Part model, mm, in its own coordinate system. Round coordinates to 2 decimals unless told otherwise and drop trailing zeros. Loops run counter-clockwise (first coordinate to the right, second up) from the corner with the lowest first, then second, coordinate; pieces in that order, holes last.
(1) Flat gauge pin, fed straight in: pin 1 (2.5 mm diameter, centred on x = 17.14, z = 43.28, fed in from +Y). Where does the tip first touch, or does it go through?
(2) Cut at C-C on y = 2.75. List the corners of the cut face in (x, z).
(3) Cut at B-B on x = 20. List the corners of the cut face in (y, z).
(4) Cut at A-A on z = 25. List the corners of the cut face in (x, y), then the cut area to 3 significant figures.
(5) Mould opens along X. For faces 1 (the face through (33, 2, 0)), 2 (the face through (0, 2, 25)), 3 (the face through (18.73, 2.03, 42.06)) say: +X half, -X half, draft (parallel to the pull), parting line (faces both ways), or undercut.
(6) Probe probe 1 along X at (y, z) = (2.9, 25); probe 2 along Z at (x, y) = (21.5, 0.7); probe 3 along X at (y, z) = (3.4, 26). List the from-to ranges inside material, lowest first.
from build123d import *

# Parameters (mm, degrees)
BOSS_EXTRUDE1_DEPTH = 50
SKETCH3_R           = 4
CUT_EXTRUDE1_DEPTH  = 10
SKETCH4_W           = 25
SKETCH4_H           = 50
CUT_EXTRUDE2_DEPTH  = 10
SKETCH6_R           = 2
CUT_EXTRUDE4_DEPTH  = 83.1035931


with BuildPart() as part:
    # Sketch2 → Boss-Extrude1 (new body)
    with BuildSketch(Plane.XY):
        Polygon((4, 4), (90, 4), (90, 0), (0, 0), (0, 4), align=None)
    extrude(amount=BOSS_EXTRUDE1_DEPTH)

    # Sketch3 → Cut-Extrude1 (cut)
    with BuildSketch(Plane(origin=(0, 4, 0), x_dir=(1, 0, 0), z_dir=(0, 1, 0))):
        with Locations(Location((20, -25, 0), (0, 0, 270))):
            Circle(SKETCH3_R)
    extrude(amount=-CUT_EXTRUDE1_DEPTH, mode=Mode.SUBTRACT)

    # Sketch4 → Cut-Extrude2 (cut)
    with BuildSketch(Plane(origin=(0, 4, 0), x_dir=(1, 0, 0), z_dir=(0, 1, 0))):
        with Locations((77.5, -25)):
            Rectangle(SKETCH4_W, SKETCH4_H)
    extrude(amount=-CUT_EXTRUDE2_DEPTH, mode=Mode.SUBTRACT)

    # Sketch6 → Cut-Extrude4 (cut, through all)
    with BuildSketch(Plane(origin=(0, 4, 0), x_dir=(1, 0, 0), z_dir=(0, 1, 0))):
        with Locations(Location((17.143662574, -43.278165567, 0), (0, 0, 180))):
            Circle(SKETCH6_R)
        with Locations(Location((22.856337427, -6.721834433, 0), (0, 0, 180))):
            Circle(SKETCH6_R)
    extrude(amount=-CUT_EXTRUDE4_DEPTH, mode=Mode.SUBTRACT)


solid = part.part
Final values:
1. pin 1: passes through
2. outline: (0, 0) - (65, 0) - (65, 50) - (0, 50) - close; hole circle Ø4 at (17.14, 43.28); hole circle Ø8 at (20, 25); hole circle Ø4 at (22.86, 6.72)
3. outline: (0, 0) - (4, 0) - (4, 21) - (0, 21) - close; (0, 29) - (4, 29) - (4, 50) - (0, 50) - close
4. outline: (0, 0) - (16, 0) - (16, 4) - (0, 4) - close; (24, 0) - (65, 0) - (65, 4) - (24, 4) - close
4. area: 228 mm2
5. face 1: draft
5. face 2: -X half
5. face 3: undercut
6. probe 1: x = 0 to 16, 24 to 65
6. probe 2: z = 0 to 5.25, 8.19 to 21.29, 28.71 to 50
6. probe 3: x = 0 to 16.13, 23.87 to 65
